from build123d import *

# Parameters (mm, degrees)
CUT_EXTRUDE1_DEPTH      = 2.54
CUT_EXTRUDE1_DEPTH_BACK = 2.54


with BuildPart() as part:
    # Sketch2 → Revolve1 (revolve)
    with BuildSketch(Plane.XY):
        with BuildLine():
            Line((0, 2.0574), (0, 1.0922))
            Line((0, 1.0922), (6.35, 1.0922))
            Line((6.35, 1.0922), (6.35, 0))
            Line((6.35, 0), (0, 0))
            Line((0, 0), (-1.7526, 0))
            add(Edge.make_bspline(
                [(0, 2.0574), (-1.7526, 2.0574), (-1.7526, 0)],
                knots=[3.141592654, 3.141592654, 3.141592654, 4.71238898, 4.71238898, 4.71238898], degree=2, weights=[1, 0.707106781, 1]))
        make_face()
    revolve(axis=Axis((6.35, 0, 0), (-1, 0, 0)))

    # 3DSketch1 → Cut-Extrude1 (cut, two sides)
    with BuildSketch(Plane(origin=(-0.762, 0.508, 0), x_dir=(-0.9284766908852594, -0.37139067635410355, 0), z_dir=(0, 0, 1))) as cut_extrude1_sk:
        Polygon((0, 0), (0.377332927, 0.943332318), (2.735663722, 0), (2.358330795, -0.943332318), align=None)
    extrude(amount=CUT_EXTRUDE1_DEPTH, mode=Mode.SUBTRACT)
    extrude(cut_extrude1_sk.sketch, amount=-CUT_EXTRUDE1_DEPTH_BACK, mode=Mode.SUBTRACT)


solid = part.part
The model under review builds one solid part; all positions refer to its coordinate system, in mm. A direction names the side the tool comes from. Coordinates: 2 decimals unless noted, no trailing zeros. Write each loop counter-clockwise with the first axis right and the second up, starting at its lowest first coordinate (ties: lowest second). Pieces come first, ordered by that corner, then holes. Notation, with made-up numbers: M 5,9 L 17,9 A15 cw 17,17 Z; hole C 7,81 d5. An arc over 180 degrees is marked long. Put each result on its own line as item: value.
1) Add section A-A on x = 4.25. Give the boundary of the cut face in (y, z).
Computed:
outline: C 0,0 d2.18
2) Clearance check with flat-ended pins moving along their axes: pin 1 Ø2 at (y, z) = (-0.5, -0.5) entering from -X; pin 2 Ø0.8 at (y, z) = (0, 1) entering from -X; pin 3 Ø0.7 at (x, z) = (-1, -0.5) entering from -Y; pin 4 Ø1 at (x, z) = (-1, 0.5) entering from +Y. State where each tip first meets the part, or that it passes through.
Computed:
pin 1: stops at x = -1.7
pin 2: stops at x = -0.76
pin 3: stops at y = -1.86
pin 4: stops at y = 1.93
3) Wall thickness on probe 1 along X at (y, z) = (0.4, 1.6); probe 2 along X at (y, z) = (0.3, 0.6); probe 3 along Z at (x, y) = (-0.25, 0.85): over which ranges is each line inside the solid? List them lowest first. Write a range as [from, to].
Computed:
probe 1: x = [-0.76, 0]
probe 2: x = [-0.76, 6.35]
probe 3: z = [-1.85, 1.85]
4) For faces 1 (the flat face through (0, 1, 1)), 2 (the flat face through (-0.762, 0, 0)), 3 (the flat face through (6.35, 0, 0)), list the 3-axis set-ups (+Z, -Z, +X, -X, +Y, -Y) from which the entire face can be reached by the end or side of a thin tool; tool diameter is ignored.
Computed:
face 1: +X
face 2: +Z, -Z, -X
face 3: +Z, -Z, +X, +Y, -Y
